Here's how the part is built. I have some questions about the finished solid (model axes, mm). Round coordinates to 2 decimals unless told otherwise and drop trailing zeros. Loops run counter-clockwise (first coordinate to the right, second up) from the corner with the lowest first, then second, coordinate; pieces in that order, holes last. Notation, with made-up numbers: M 9.5,56 L 39.5,56 A18 cw 39.5,71 Z; hole C 79.25,66.25 d4. An arc over 180 degrees is marked long. Use a Markdown table: item, result.
```python
from build123d import *

# Parameters (mm, degrees)
F0_R     = 7.1501
F0_R_2   = 2.3876
F1_DEPTH = 3.175


with BuildPart() as f1:
    # F0 (on Top) → F1 (new body)
    with BuildSketch(Plane.XY):
        Circle(F0_R)
        with BuildLine():
            ThreePointArc((4.287339, 2.073676), (4.399976, 1.82253), (4.497917, 1.565296))
            ThreePointArc((4.497917, 1.565296), (5.787227, 1.212473), (6.35, 0))
            ThreePointArc((6.35, 0), (5.787227, -1.212473), (4.497917, -1.565296))
            ThreePointArc((4.497917, -1.565296), (0, -4.7625), (-4.497917, -1.565296))
            ThreePointArc((-4.497917, -1.565296), (-6.35, 0), (-4.497917, 1.565296))
            ThreePointArc((-4.497917, 1.565296), (-4.399976, 1.82253), (-4.287339, 2.073676))
            ThreePointArc((-4.287339, 2.073676), (-4.490128, 4.490128), (-2.073676, 4.287339))
            ThreePointArc((-2.073676, 4.287339), (-1.628125, 4.475558), (-1.165781, 4.617614))
            ThreePointArc((-1.165781, 4.617614), (-0.072582, 5.935006), (1.17475, 4.7625))
            ThreePointArc((1.17475, 4.7625), (1.172506, 4.689918), (1.165781, 4.617614))
            ThreePointArc((1.165781, 4.617614), (1.628125, 4.475558), (2.073676, 4.287339))
            ThreePointArc((2.073676, 4.287339), (3.850327, 4.879921), (4.955096, 3.367596))
            ThreePointArc((4.955096, 3.367596), (4.778314, 2.639563), (4.287339, 2.073676))
        make_face(mode=Mode.SUBTRACT)
        with BuildLine():
            ThreePointArc((4.497917, -1.565296), (3.175, 0), (4.497917, 1.565296))
            ThreePointArc((4.497917, 1.565296), (4.399976, 1.82253), (4.287339, 2.073676))
            ThreePointArc((4.287339, 2.073676), (2.245064, 2.245064), (2.073676, 4.287339))
            ThreePointArc((2.073676, 4.287339), (1.628125, 4.475558), (1.165781, 4.617614))
            ThreePointArc((1.165781, 4.617614), (0, 3.58775), (-1.165781, 4.617614))
            ThreePointArc((-1.165781, 4.617614), (-1.628125, 4.475558), (-2.073676, 4.287339))
            ThreePointArc((-2.073676, 4.287339), (-1.855271, 3.850327), (-1.780096, 3.367596))
            ThreePointArc((-1.780096, 3.367596), (-2.639563, 1.956879), (-4.287339, 2.073676))
            ThreePointArc((-4.287339, 2.073676), (-4.399976, 1.82253), (-4.497917, 1.565296))
            ThreePointArc((-4.497917, 1.565296), (-3.550027, 1.024727), (-3.175, 0))
            ThreePointArc((-3.175, 0), (-3.550027, -1.024727), (-4.497917, -1.565296))
            ThreePointArc((-4.497917, -1.565296), (0, -4.7625), (4.497917, -1.565296))
        make_face()
        Circle(F0_R_2, mode=Mode.SUBTRACT)
    extrude(amount=F1_DEPTH)


solid = f1.part
```
Q1. Will these pins go through, and if not, where does the flat tip stop? P1, Ø1, axis at x = -0.5, z = 1.5, coming from the -Y side; P2, Ø1, axis at y = -4, z = 0.5, coming from the +X side; P3, Ø1, axis at y = 3, z = 1, coming from the +X side.
Return value:
| item | result |
|---|---|
| P1 | stops at y = -7.15 |
| P2 | stops at x = 6.23 |
| P3 | stops at x = 6.7 |
Q2. Imagine slicing it at D-D, the plane y = 0.5. Please give me the cut outline in (x, z) (3 decimals), then the cut area to 3 significant figures.
Return value:
| item | result |
|---|---|
| outline | M -7.133,0 L -6.269,0 L -6.269,3.175 L -7.133,3.175 Z; M -3.256,0 L -2.335,0 L -2.335,3.175 L -3.256,3.175 Z; M 2.335,0 L 3.256,0 L 3.256,3.175 L 2.335,3.175 Z; M 6.269,0 L 7.133,0 L 7.133,3.175 L 6.269,3.175 Z |
| area | 11.3 mm^2 |
Q3. Imagine slicing it at B-B, the plane x = 0. Please give me the cut outline in (y, z) (3 decimals), then the cut area to 3 significant figures.
Return value:
| item | result |
|---|---|
| outline | M -7.15,0 L -2.388,0 L -2.388,3.175 L -7.15,3.175 Z; M 2.388,0 L 3.588,0 L 3.588,3.175 L 2.388,3.175 Z; M 5.937,0 L 7.15,0 L 7.15,3.175 L 5.937,3.175 Z |
| area | 22.8 mm^2 |
Q4. Imagine slicing it at C-C, the plane x = -3. Please give me the cut outline in (y, z) (3 decimals).
Return value:
| item | result |
|---|---|
| outline | M -6.49,0 L 1.823,0 L 1.823,3.175 L -6.49,3.175 Z; M 4.912,0 L 6.49,0 L 6.49,3.175 L 4.912,3.175 Z |
Q5. Imagine slicing it at A-A, the plane z = 2.35. Give the number of separate pieces and of enclosed holes in the cut face, then the cut area to 3 significant figures.
Return value:
| item | result |
|---|---|
| separate pieces | 1 |
| enclosed holes | 6 |
| area | 107 mm^2 |
Q6. We'd pull the mould along Y, two halves only. Please class faces 1 (the cylindrical face through (-1.55, -6.98, 1.57)), 2 (the flat face through (0, -3, 0)), 3 (the cylindrical face through (-0.52, -2.33, 1.57)): pulls with the +Y half, pulls with the -Y half, needs draft (parallel to the pull), parting line crosses it, or undercut.
Return value:
| item | result |
|---|---|
| face 1 | parting line crosses it |
| face 2 | needs draft |
| face 3 | undercut |
Q7. I need wall thicknesses on line 1 (Y direction, x = 0, z = 2.05); line 2 (Y direction, x = 0.75, z = 2.6); line 3 (X direction, y = -1.25, z = 2.7). Which ranges of each line are inside material? Lowest first, please. Write a range as from..to.
Return value:
| item | result |
|---|---|
| line 1 | y = -7.15..-2.39, 2.39..3.59, 5.94..7.15 |
| line 2 | y = -7.11..-2.27, 2.27..3.86, 5.67..7.11 |
| line 3 | x = -7.04..-5.74, -3.78..-2.03, 2.03..3.78, 5.74..7.04 |
